from build123d import *

# Parameters (mm, degrees)
BOSS_EXTRUDE1_DEPTH = 60
SKETCH3_R           = 15.895839237
CUT_EXTRUDE1_DEPTH  = 10
SKETCH4_R           = 3
CUT_EXTRUDE2_DEPTH  = 40


with BuildPart() as part:
    # Sketch2 → Boss-Extrude1 (new body)
    with BuildSketch(Plane.XY):
        with BuildLine():
            Line((-18.5, -41.5), (18.5, -41.5))
            ThreePointArc((18.5, -41.5), (21.328427125, -40.328427125), (22.5, -37.5))
            Line((22.5, -37.5), (22.5, 37.5))
            ThreePointArc((22.5, 37.5), (21.328427125, 40.328427125), (18.5, 41.5))
            Line((18.5, 41.5), (-18.5, 41.5))
            ThreePointArc((-18.5, 41.5), (-21.328427125, 40.328427125), (-22.5, 37.5))
            Line((-22.5, 37.5), (-22.5, -37.5))
            ThreePointArc((-22.5, -37.5), (-21.328427125, -40.328427125), (-18.5, -41.5))
        make_face()
    extrude(amount=BOSS_EXTRUDE1_DEPTH)

    # Sketch3 → Cut-Extrude1 (cut)
    with BuildSketch(Plane.XY.offset(60)):
        Circle(SKETCH3_R)
    extrude(amount=-CUT_EXTRUDE1_DEPTH, mode=Mode.SUBTRACT)

    # Sketch4 → Cut-Extrude2 (cut)
    with BuildSketch(Plane.XY.offset(50)):
        with Locations((7.338844811, 6.864557304)):
            Circle(SKETCH4_R)
        with Locations((-5.644149057, 6.864557304)):
            Circle(SKETCH4_R)
        with Locations((0, -5.510422777)):
            Circle(SKETCH4_R)
    extrude(amount=-CUT_EXTRUDE2_DEPTH, mode=Mode.SUBTRACT)


solid = part.part
Geometry check sheet. Reference: the model listing, model coordinates, mm. A direction names the side the tool comes from. Round coordinates to 2 decimals unless told otherwise and drop trailing zeros. Write each loop counter-clockwise with the first axis right and the second up, starting at its lowest first coordinate (ties: lowest second). Pieces come first, ordered by that corner, then holes.
Item 1: Section check B-B (y = 0). Record the boundary of the cut face in (x, z), plus the area to 3 significant figures.
Determined:
outline: (-22.5, 0) - (22.5, 0) - (22.5, 60) - (15.9, 60) - (15.9, 50) - (-15.9, 50) - (-15.9, 60) - (-22.5, 60) - close
area: 2,380 mm2
Item 2: Section check C-C (z = 30). Record the boundary of the cut face in (x, y).
Determined:
outline: (-22.5, -37.5) arc R4 ccw to (-18.5, -41.5) - (18.5, -41.5) arc R4 ccw to (22.5, -37.5) - (22.5, 37.5) arc R4 ccw to (18.5, 41.5) - (-18.5, 41.5) arc R4 ccw to (-22.5, 37.5) - close; hole circle Ø6 at (-5.64, 6.86); hole circle Ø6 at (0, -5.51); hole circle Ø6 at (7.34, 6.86)
Item 3: Go/stop test with flat-tipped pins: pin 1 Ø2 at (x, y) = (-14.5, -1.5) entering from +Z; pin 2 Ø2 at (x, y) = (-13, 24) entering from -Z; pin 3 Ø1.8 at (x, y) = (-6, 6) entering from +Z. Record where each tip stops, or that it passes through.
Determined:
pin 1: stops at z = 50
pin 2: stops at z = 0
pin 3: stops at z = 10
Item 4: Section check D-D (x = -13.5). Record the boundary of the cut face in (y, z).
Determined:
outline: (-41.5, 0) - (41.5, 0) - (41.5, 60) - (8.39, 60) - (8.39, 50) - (-8.39, 50) - (-8.39, 60) - (-41.5, 60) - close
Item 5: Section check A-A (x = 0). Record the boundary of the cut face in (y, z).
Determined:
outline: (-41.5, 0) - (41.5, 0) - (41.5, 60) - (15.9, 60) - (15.9, 50) - (-2.51, 50) - (-2.51, 10) - (-8.51, 10) - (-8.51, 50) - (-15.9, 50) - (-15.9, 60) - (-41.5, 60) - close
Item 6: Mould release check, pull along Y, two halves, no side actions. Record for faces 3 (the face through (0, -5, 10)), 4 (the face through (21.297, -40.359, 29.58)), 5 (the face through (-2.997, -5.379, 30.28)), 6 (the face through (22.5, -1, 30)): +Y half, -Y half, draft (parallel to the pull), parting line (faces both ways), or undercut.
Determined:
face 3: undercut
face 4: -Y half
face 5: undercut
face 6: draft
Item 7: Access from +Z, -Z, +X, -X, +Y, -Y to the whole of each face (thin tool, end or side, straight path). Record for faces 1 (the face through (-22.5, 1, 30)), 2 (the face through (8.72, 4.2, 30.28)).
Determined:
face 1: +Z, -Z, -X, +Y, -Y
face 2: +Z
Item 8: Material ranges on line 1 along Y through (x, z) = (0, 34); line 2 along Y through (x, z) = (-5.5, 44); line 3 along Y through (x, z) = (20.5, 48.5), recorded low to high.
Determined:
line 1: y = -41.5 to -8.51, -2.51 to 41.5
line 2: y = -41.5 to 3.87, 9.86 to 41.5
line 3: y = -40.96 to 40.96
